Geometry check sheet. Reference: the model listing, model coordinates, mm. A direction names the side the tool comes from. Round coordinates to 2 decimals unless told otherwise and drop trailing zeros. Order: outer loops, then holes, each group sorted by start corner. A loop starts at its lowest first (then second) coordinate and runs counter-clockwise, first axis right, second up.
(1) Thickness scan on L1, parallel to Y at x = 30, z = 180.5; L2, parallel to Z at x = 10, y = 6.75; L3, parallel to Y at x = 5, z = 117.5. Record the ranges inside material, lowest first.
(2) Draft check along Z on faces 1 (the face through (9.46, 6.9, 37.56)), 2 (the face through (30, 12, 25)), 3 (the face through (30, 96, 178)), 4 (the face through (12.5, 6.9, 30.16)). Enter one of: pulls with the +Z half, pulls with the -Z half, needs draft (parallel to the pull), parting line crosses it, or undercut.
(3) Gauge pin test, flat ends, axial feed: P1, Ø0.9, axis at x = 25.5, z = 176, coming from the -Y side; P2, Ø4, axis at x = 23.5, y = 69.5, coming from the -Z side; P3, Ø20, axis at x = 24, z = 92, coming from the +Y side; P4, Ø4, axis at x = 30, z = 20, coming from the -Y side. Record the tip position at first contact, or that the pin passes through.
(4) Set-up check for faces 5 (the face through (22, 6, 30)), 6 (the face through (30, 76, 175)), 7 (the face through (10, 14, 25)), 8 (the face through (30, 36, 175)): record each of +Z, -Z, +X, -X, +Y, -Y from which the full face is reachable in a straight line by a thin tool's end or side.
(5) Cross-section at D-D on x = 18. Enter the section's corners in (y, z).
(6) Cross-section at A-A on z = 172. Enter the section's corners in (x, y).
(7) Cross-section at C-C on z = 40. Enter the section's corners in (x, y), and give its area (3 significant figures).
(8) Cross-section at B-B on x = 9.5. Enter the section's corners in (y, z).
from build123d import *

# Parameters (mm, degrees)
F0_W      = 40
F0_H      = 16
F1_DEPTH  = 190
F2_R      = 2.5
F3_DEPTH  = 20
F4_W      = 40
F4_H      = 50
F5_DEPTH  = 2
F6_W      = 20
F6_H      = 50
F7_DEPTH  = 2
F8_R      = 1
F9_DEPTH  = 20
F10_W     = 10
F10_H     = 75
F11_DEPTH = 100
F13_DEPTH = 10
F14_W     = 20
F14_H     = 5
F15_DEPTH = 3
F17_DEPTH = 15


with BuildPart() as f1:
    # F0 (on Top) → F1 (new body)
    with BuildSketch(Plane.XY):
        with Locations((20, 8)):
            Rectangle(F0_W, F0_H)
    extrude(amount=F1_DEPTH)

    # F2 (on face) → F3 (cut)
    with BuildSketch(Plane.XZ):
        with Locations((10, 40)):
            Circle(F2_R)
        with Locations((30, 40)):
            Circle(F2_R)
        with Locations((10, 20)):
            Circle(F2_R)
        with Locations((30, 20)):
            Circle(F2_R)
        with BuildLine():
            ThreePointArc((20, 37.5), (12.5, 30), (20, 22.5))
            Line((20, 22.5), (22, 22.5))
            Line((22, 22.5), (22, 37.5))
            Line((22, 37.5), (20, 37.5))
        make_face()
    extrude(amount=-F3_DEPTH, mode=Mode.SUBTRACT)

    # F4 (on face) → F5 (cut)
    with BuildSketch(Plane(origin=(0, 16, 0), x_dir=(-1, 0, 0), z_dir=(0, 1, 0))):
        with Locations((-20, 25)):
            Rectangle(F4_W, F4_H)
    extrude(amount=-F5_DEPTH, mode=Mode.SUBTRACT)

    # F6 (on face) → F7 (cut)
    with BuildSketch(Plane(origin=(0, 14, 0), x_dir=(-1, 0, 0), z_dir=(0, 1, 0))):
        with Locations((-30, 25)):
            Rectangle(F6_W, F6_H)
    extrude(amount=-F7_DEPTH, mode=Mode.SUBTRACT)

    # F8 (on face) → F9 (cut)
    with BuildSketch(Plane.XY.offset(190)):
        with Locations((30, 12)):
            Circle(F8_R)
        with Locations((30, 4)):
            Circle(F8_R)
    extrude(amount=-F9_DEPTH, mode=Mode.SUBTRACT)

    # F10 (on face) → F11 (join)
    with BuildSketch(Plane(origin=(0, 16, 0), x_dir=(-1, 0, 0), z_dir=(0, 1, 0))):
        Polygon((-20, 190), (-40, 190), (-40, 175), (-35, 175), (-25, 175), (-20, 175), align=None)
        with Locations((-30, 137.5)):
            Rectangle(F10_W, F10_H)
    extrude(amount=F11_DEPTH)

    # F12 (on face) → F13 (cut)
    with BuildSketch(Plane(origin=(25, 0, 0), x_dir=(0, -1, 0), z_dir=(-1, 0, 0))):
        with BuildLine():
            ThreePointArc((-116, 170.7106781187), (-134.3012701892, 38.7627564304), (-16, 100))
            ThreePointArc((-16, 100), (-37.966991411, 153.033008589), (-91, 175))
            Line((-91, 175), (-91, 100))
            Line((-91, 100), (-116, 100))
            Line((-116, 100), (-116, 170.7106781187))
        make_face()
        with BuildLine():
            Line((-91, 100), (-91, 175))
            ThreePointArc((-91, 175), (-103.6826484044, 173.919891974), (-116, 170.7106781187))
            Line((-116, 170.7106781187), (-116, 100))
            Line((-116, 100), (-91, 100))
        make_face()
        with BuildLine():
            ThreePointArc((-116, 170.7106781187), (-103.6826484044, 173.919891974), (-91, 175))
            Line((-91, 175), (-116, 175))
            Line((-116, 175), (-116, 170.7106781187))
        make_face()
    extrude(amount=-F13_DEPTH, mode=Mode.SUBTRACT)

    # F14 (on face) → F15 (cut)
    with BuildSketch(Plane(origin=(0, 0, 175), x_dir=(1, 0, 0), z_dir=(0, 0, -1))):
        with Locations((30, -96)):
            Rectangle(F14_W, F14_H)
        with Locations((30, -76)):
            Rectangle(F14_W, F14_H)
        with Locations((30, -56)):
            Rectangle(F14_W, F14_H)
        with Locations((30, -36)):
            Rectangle(F14_W, F14_H)
    extrude(amount=-F15_DEPTH, mode=Mode.SUBTRACT)

    # F16 (on face) → F17 (join)
    with BuildSketch(Plane.XY.offset(190)):
        with BuildLine():
            ThreePointArc((20, 36), (14.1421356237, 21.8578643763), (0, 16))
            Line((0, 16), (20, 16))
            Line((20, 16), (20, 36))
        make_face()
    extrude(amount=-F17_DEPTH)


solid = f1.part
Found:
1. L1: y = 0 to 3, 5 to 11, 13 to 116
1. L2: z = 0 to 17.5, 22.5 to 37.5, 42.5 to 190
1. L3: y = 0 to 16
2. face 1: undercut
2. face 2: needs draft
2. face 3: pulls with the -Z half
2. face 4: undercut
3. P1: stops at y = 0
3. P2: stops at z = 171.44
3. P3: stops at y = 16.03
3. P4: passes through
4. face 5: +Y, -Y
4. face 6: +X, -X
4. face 7: -Z, +X, -X, +Y
4. face 8: +X
5. outline: (0, 0) - (14, 0) - (14, 22.77) - (0, 22.77) - close; (0, 37.23) - (14, 37.23) - (14, 50) - (16, 50) - (16, 175) - (27.28, 175) - (27.28, 190) - (0, 190) - close
6. outline: (0, 0) - (40, 0) - (40, 16) - (35, 16) - (35, 70) - (25, 70) - (25, 16) - (0, 16) - close; hole circle Ø2 at (30, 4); hole circle Ø2 at (30, 12)
7. outline: (0, 0) - (7.5, 0) - (7.5, 14) - (0, 14) - close; (12.5, 0) - (27.5, 0) - (27.5, 12) - (20, 12) - (20, 14) - (12.5, 14) - close; (32.5, 0) - (40, 0) - (40, 12) - (32.5, 12) - close
7. area: 390 mm2
8. outline: (0, 0) - (14, 0) - (14, 17.55) - (0, 17.55) - close; (0, 22.45) - (14, 22.45) - (14, 37.55) - (0, 37.55) - close; (0, 42.45) - (14, 42.45) - (14, 50) - (16, 50) - (16, 175) - (18.4, 175) - (18.4, 190) - (0, 190) - close
